from build123d import *

# Parameters (mm, degrees)
SKETCH1_R          = 34.925
EXTRUDE1_DEPTH     = 12.7
SKETCH3_R          = 3.3655
CUT_EXTRUDE2_DEPTH = 12.7
CIRPATTERN1_COUNT  = 6


with BuildPart() as part:
    # Sketch1 → Extrude1 (new body)
    with BuildSketch(Plane(origin=(0, 0, 0), x_dir=(1, 0, 0), z_dir=(0, 1, 0))):
        Circle(SKETCH1_R)
    extrude(amount=EXTRUDE1_DEPTH)

    # Sketch3 → Cut-Extrude2 (cut)
    with BuildSketch(Plane(origin=(0, 0, 0), x_dir=(1, 0, 0), z_dir=(0, 1, 0))):
        with Locations((0, 29.337)):
            Circle(SKETCH3_R)
    cut_extrude2 = extrude(amount=CUT_EXTRUDE2_DEPTH, mode=Mode.SUBTRACT)

    # CirPattern1: Cut-Extrude2 ×6 about axis
    cirpattern1_axis = Axis((0, 0, 0), (0, 1, 0))
    for i in range(1, CIRPATTERN1_COUNT):
        add(cut_extrude2.rotate(cirpattern1_axis, i * 360 / CIRPATTERN1_COUNT), mode=Mode.SUBTRACT)


solid = part.part
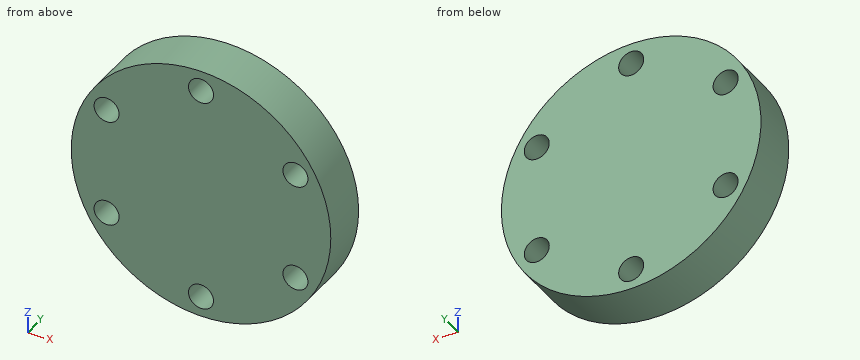
Source: CAD feature listing. Evaluate the final solid. Frame: model axes, mm. Coordinates: 2 decimals unless noted, no trailing zeros. Loops run counter-clockwise (first coordinate to the right, second up) from the corner with the lowest first, then second, coordinate; pieces in that order, holes last. Notation, with made-up numbers: (33, -31) - (84, -31) arc R5 ccw to (84, -26) - close; hole circle Ø7 at (24, 83). An arc over 180 degrees is marked (long way). One line per question, with ' | ' between items.
1) Section A-A, the plane x = 0. Return loops of the section in (y, z) (1 decimal), then the cut area to 3 significant figures.
Report:
outline: (0, -34.9) - (12.7, -34.9) - (12.7, -32.7) - (0, -32.7) - close; (0, -26) - (12.7, -26) - (12.7, 26) - (0, 26) - close; (0, 32.7) - (12.7, 32.7) - (12.7, 34.9) - (0, 34.9) - close | area: 716 mm²
2) Line query: line 1 along X through (y, z) = (12, -13); line 2 along Z through (x, y) = (1.5, 7); line 3 along X through (y, z) = (2.5, 16). Output: solid intervals per line, ascending.
Report:
line 1: x = -32.42 to -28.33, -22.48 to 22.48, 28.33 to 32.42 | line 2: z = -34.89 to -32.35, -26.32 to 26.32, 32.35 to 34.89 | line 3: x = -31.04 to -28.5, -22.32 to 22.32, 28.5 to 31.04
3) First-contact query: P1, Ø5, axis at y = 7, z = -3, coming from the +X side; P2, Ø2, axis at y = 11, z = 21, coming from the -X side. Flat tips, straight axial feed; report the tip coordinate or a pass-through.
Report:
P1: stops at x = 34.92 | P2: stops at x = -28.63
4) Section C-C, the plane y = 4.75. Give the number of separate pieces and of enclosed holes in the cut face, then the cut area to 3 significant figures.
Report:
separate pieces: 1 | enclosed holes: 6 | area: 3,620 mm²
5) Section D-D, the plane z = 6.5. Return loops of the section in (x, y), then the cut area to 3 significant figures.
Report:
outline: (-34.31, 0) - (34.31, 0) - (34.31, 12.7) - (-34.31, 12.7) - close | area: 872 mm²
6) Section B-B, the plane z = 16. Return loops of the section in (x, y), then the cut area to 3 significant figures.
Report:
outline: (-31.04, 0) - (-28.5, 0) - (-28.5, 12.7) - (-31.04, 12.7) - close; (-22.32, 0) - (22.32, 0) - (22.32, 12.7) - (-22.32, 12.7) - close; (28.5, 0) - (31.04, 0) - (31.04, 12.7) - (28.5, 12.7) - close | area: 632 mm²
